Design review of the part built by this model. Coordinates are the model's own, in mm. A direction names the side the tool comes from. Round coordinates to 2 decimals unless told otherwise and drop trailing zeros. Loops run counter-clockwise (first coordinate to the right, second up) from the corner with the lowest first, then second, coordinate; pieces in that order, holes last. Notation, with made-up numbers: (13, 25.25) - (56, 25.25) arc R32 ccw to (56, 56.25) - close; hole circle Ø5 at (-8, -30.75). An arc over 180 degrees is marked (long way). Return JSON: item names as keys, results as strings. Group by question number.
(1) We need section D-D, the plane x = 9.25. Write out the cut boundary in (y, z) (3 decimals), and give its area (3 significant figures).
(2) We need section B-B, the plane x = 0. Write out the cut boundary in (y, z) (3 decimals).
(3) The part is to be moulded in two halves that separate along Y. For faces 1 (the flat face through (0, 12.7, 2)), 2 (the flat face through (0, -3.175, 8)), 3 (the flat face through (6.35, 0, 13)), 4 (the cylindrical face through (-10.15, 7.924, 2.191)), say which applies: pulls with the +Y half, pulls with the -Y half, needs draft (parallel to the pull), parting line crosses it, or undercut.
(4) We need section A-A, the plane z = 4. Write out the cut boundary in (x, y) (1 decimal).
(5) For faces 5 (the flat face through (0, 6.35, 13)), 6 (the flat face through (-6.35, 0, 13)), 7 (the flat face through (0, 3.175, 8)), 8 (the flat face through (4, 0, 10.795)), 9 (the flat face through (3.175, 0, 8)), list the 3-axis set-ups (+Z, -Z, +X, -X, +Y, -Y) from which the entire face can be reached by the end or side of a thin tool; tool diameter is ignored.
(6) Clearance check with flat-ended pins moving along their axes: pin 1 (4 mm diameter, centred on x = 0, z = 13, fed in from -Y); pin 2 (3 mm diameter, centred on x = -0.5, z = 6.5, fed in from -Y) (3 decimals); pin 3 (5.5 mm diameter, centred on y = -1.5, z = 13.5, fed in from -X); pin 4 (3 mm diameter, centred on x = -4.5, y = 10, fed in from -Z). State where each tip first meets the part, or that it passes through.
(7) Wall thickness on L1, parallel to Y at x = -8.89, z = 1.75; L2, parallel to Z at x = 6, y = -2.25 (3 decimals); L3, parallel to Y at x = -8.5, z = 3: over which ranges is each line inside the solid? List them lowest first. Write a range as [from, to].
(8) We need section C-C, the plane y = 8.5. Write out the cut boundary in (x, z) (3 decimals), and give its area (3 significant figures).
from build123d import *

# Parameters (mm, degrees)
F0_R     = 1.5875
F1_DEPTH = 4.445
F2_W     = 6.35
F2_H     = 6.35
F3_DEPTH = 6.35
F4_W     = 12.7
F4_H     = 12.7
F5_DEPTH = 5.08


with BuildPart() as f1:
    # F0 (on Top) → F1 (new body)
    with BuildSketch(Plane.XY):
        with BuildLine():
            ThreePointArc((12.7, 8.89), (11.584077, 11.584077), (8.89, 12.7))
            Line((8.89, 12.7), (-8.89, 12.7))
            ThreePointArc((-8.89, 12.7), (-11.584077, 11.584077), (-12.7, 8.89))
            Line((-12.7, 8.89), (-12.7, -8.89))
            ThreePointArc((-12.7, -8.89), (-11.584077, -11.584077), (-8.89, -12.7))
            Line((-8.89, -12.7), (8.89, -12.7))
            ThreePointArc((8.89, -12.7), (11.584077, -11.584077), (12.7, -8.89))
            Line((12.7, -8.89), (12.7, 8.89))
        make_face()
        with Locations((-8.89, -8.89)):
            Circle(F0_R, mode=Mode.SUBTRACT)
        with Locations((8.89, -8.89)):
            Circle(F0_R, mode=Mode.SUBTRACT)
        with Locations((-8.89, 8.89)):
            Circle(F0_R, mode=Mode.SUBTRACT)
        with Locations((8.89, 8.89)):
            Circle(F0_R, mode=Mode.SUBTRACT)
    extrude(amount=F1_DEPTH)

    # F2 (on face) → F3 (join)
    with BuildSketch(Plane.XY.offset(4.445)):
        Rectangle(F2_W, F2_H)
    extrude(amount=F3_DEPTH)

    # F4 (on face) → F5 (join)
    with BuildSketch(Plane.XY.offset(10.795)):
        Rectangle(F4_W, F4_H)
    extrude(amount=F5_DEPTH)


solid = f1.part
Solutions:
{
 "1": {"outline": "(-12.683, 0) - (-10.436, 0) - (-10.436, 4.445) - (-12.683, 4.445) - close; (-7.344, 0) - (7.344, 0) - (7.344, 4.445) - (-7.344, 4.445) - close; (10.436, 0) - (12.683, 0) - (12.683, 4.445) - (10.436, 4.445) - close", "area": "85.3 mm^2"},
 "2": {"outline": "(-12.7, 0) - (12.7, 0) - (12.7, 4.445) - (3.175, 4.445) - (3.175, 10.795) - (6.35, 10.795) - (6.35, 15.875) - (-6.35, 15.875) - (-6.35, 10.795) - (-3.175, 10.795) - (-3.175, 4.445) - (-12.7, 4.445) - close"},
 "3": {"face 1": "pulls with the +Y half", "face 2": "pulls with the -Y half", "face 3": "needs draft", "face 4": "undercut"},
 "4": {"outline": "(-12.7, -8.9) arc R3.8 ccw to (-8.9, -12.7) - (8.9, -12.7) arc R3.8 ccw to (12.7, -8.9) - (12.7, 8.9) arc R3.8 ccw to (8.9, 12.7) - (-8.9, 12.7) arc R3.8 ccw to (-12.7, 8.9) - close; hole circle Ø3.2 at (-8.9, -8.9); hole circle Ø3.2 at (-8.9, 8.9); hole circle Ø3.2 at (8.9, -8.9); hole circle Ø3.2 at (8.9, 8.9)"},
 "5": {"face 5": "+Z, +X, -X, +Y", "face 6": "+Z, -X, +Y, -Y", "face 7": "+X, -X, +Y", "face 8": "none", "face 9": "+X, +Y, -Y"},
 "6": {"pin 1": "y = -6.35", "pin 2": "y = -3.175", "pin 3": "x = -6.35", "pin 4": "z = 0"},
 "7": {"L1": "[-12.7, -10.48], [-7.3, 7.3], [10.48, 12.7]", "L2": "[0, 4.445], [10.795, 15.875]", "L3": "[-12.7, -10.43], [-7.35, 7.35], [10.43, 12.7]"},
 "8": {"outline": "(-12.7, 0) - (-10.429, 0) - (-10.429, 4.445) - (-12.7, 4.445) - close; (-7.351, 0) - (7.351, 0) - (7.351, 4.445) - (-7.351, 4.445) - close; (10.429, 0) - (12.7, 0) - (12.7, 4.445) - (10.429, 4.445) - close", "area": "85.5 mm^2"}
}
